from build123d import *

# Parameters (mm, degrees)
CROQUIS1_W              = 20
CROQUIS1_H              = 20
SALIENTE_EXTRUIR1_DEPTH = 16
CROQUIS2_R              = 5
CROQUIS2_R_2            = 2.25
SALIENTE_EXTRUIR2_DEPTH = 10
CROQUIS6_R              = 7.5
CROQUIS6_R_2            = 6.35
SALIENTE_EXTRUIR3_DEPTH = 15
CROQUIS7_R              = 2.25
CORTAR_EXTRUIR1_DEPTH   = 10


with BuildPart() as part:
    # Croquis1 → Saliente-Extruir1 (new body)
    with BuildSketch(Plane.XY):
        Rectangle(CROQUIS1_W, CROQUIS1_H)
    extrude(amount=SALIENTE_EXTRUIR1_DEPTH)

    # Croquis2 → Saliente-Extruir2 (add)
    with BuildSketch(Plane.XY.offset(16)):
        Circle(CROQUIS2_R)
        Circle(CROQUIS2_R_2, mode=Mode.SUBTRACT)
    extrude(amount=SALIENTE_EXTRUIR2_DEPTH)

    # Croquis6 → Saliente-Extruir3 (add)
    with BuildSketch(Plane(origin=(0, 10, 0), x_dir=(1, 0, 0), z_dir=(0, 1, 0))):
        with Locations(Location((0, -8, 0), (0, 0, 270))):
            Circle(CROQUIS6_R)
        with Locations(Location((0, -8, 0), (0, 0, 270))):
            Circle(CROQUIS6_R_2, mode=Mode.SUBTRACT)
    extrude(amount=SALIENTE_EXTRUIR3_DEPTH)

    # Croquis7 → Cortar-Extruir1 (cut)
    with BuildSketch(Plane(origin=(0, 10, 0), x_dir=(1, 0, 0), z_dir=(0, 1, 0))):
        with Locations(Location((0, -20, 0), (0, 0, 270))):
            Circle(CROQUIS7_R)
    extrude(amount=-CORTAR_EXTRUIR1_DEPTH, mode=Mode.SUBTRACT)


solid = part.part
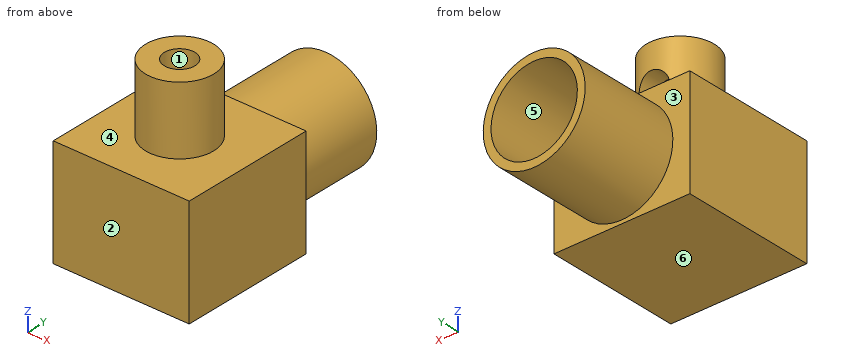
Read the model definition and answer for the solid it produces. Units are mm, in the model's axes. Face numbers are marked on the shaded views. A direction names the side the tool comes from. Coordinates: 2 decimals unless noted, no trailing zeros. Loops run counter-clockwise (first coordinate to the right, second up) from the corner with the lowest first, then second, coordinate; pieces in that order, holes last. Notation, with made-up numbers: (13, -1) -> (36, -1) arc R22 cw to (36, 19) -> close; hole circle Ø3 at (16.25, 62.25). An arc over 180 degrees is marked (long way). Write item = value, one per line. Start each with the question number.
1) The part is cut by section B-B, the plane z = 8. Determine the outline of the cut face in (x, y), plus the area to 4 significant figures.
2) For the marked faces 1, 2 and 3, determine the directions among +Z, -Z, +X, -X, +Y, -Y from which every point of the face is accessible in a straight line to the end or side of a thin tool.
3) The part is cut by section C-C, the plane y = 22. Determine the outline of the cut face in (x, z), plus the area to 3 significant figures.
4) Find the intervals of material crossed by L1, parallel to Z at x = 0, y = 2.85; L2, parallel to X at y = 15.5, z = 8; L3, parallel to X at y = 3.7, z = 20, in increasing order. Write a range as from..to.
5) The mould has two halves that part along Z. Classify the marked faces 4, 5 and 6: pulls with the +Z half, pulls with the -Z half, needs draft (parallel to the pull), parting line crosses it, or undercut.
6) Given P1, Ø4, axis at x = -2, z = 9, coming from the +Y side; P2, Ø3.5, axis at x = 0, z = 20, coming from the +Y side, each flat-ended and moving along its own axis, determine where each tip first touches the part or whether it passes through.
7) The part is cut by section A-A, the plane x = 0. Determine the outline of the cut face in (y, z), plus the area to 3 significant figures.
8) The part is cut by section D-D, the plane x = 3. Determine the outline of the cut face in (y, z), plus the area to 3 significant figures.
Result:
q1.outline = (-10, -10) -> (10, -10) -> (10, 10) -> (7.5, 10) -> (7.5, 25) -> (6.35, 25) -> (6.35, 10) -> (-6.35, 10) -> (-6.35, 25) -> (-7.5, 25) -> (-7.5, 10) -> (-10, 10) -> close
q1.area = 434.5 mm²
q2.face_1 = +Z
q2.face_2 = +Z, -Z, +X, -X, -Y
q2.face_3 = +Y
q3.outline = circle Ø15 at (0, 8); hole circle Ø12.7 at (0, 8)
q3.area = 50.0 mm²
q4.L1 = 0..17.75, 22.25..26
q4.L2 = -7.5..-6.35, 6.35..7.5
q4.L3 = -3.36..-2.25, 2.25..3.36
q5.face_4 = pulls with the +Z half
q5.face_5 = undercut
q5.face_6 = pulls with the -Z half
q6.P1 = 10
q6.P2 = -1.41
q7.outline = (-10, 0) -> (10, 0) -> (10, 0.5) -> (25, 0.5) -> (25, 1.65) -> (10, 1.65) -> (10, 14.35) -> (25, 14.35) -> (25, 15.5) -> (10, 15.5) -> (10, 16) -> (5, 16) -> (5, 17.75) -> (2.25, 17.75) -> (2.25, 16) -> (-2.25, 16) -> (-2.25, 26) -> (-5, 26) -> (-5, 16) -> (-10, 16) -> close; (2.25, 22.25) -> (5, 22.25) -> (5, 26) -> (2.25, 26) -> close
q7.area = 397 mm²
q8.outline = (-10, 0) -> (10, 0) -> (10, 1.13) -> (25, 1.13) -> (25, 2.4) -> (10, 2.4) -> (10, 13.6) -> (25, 13.6) -> (25, 14.87) -> (10, 14.87) -> (10, 16) -> (4, 16) -> (4, 26) -> (-4, 26) -> (-4, 16) -> (-10, 16) -> close
q8.area = 438 mm²
